Here's how the part is built. I have some questions about the finished solid (model axes, mm). A direction names the side the tool comes from. Round coordinates to 2 decimals unless told otherwise and drop trailing zeros. Loops run counter-clockwise (first coordinate to the right, second up) from the corner with the lowest first, then second, coordinate; pieces in that order, holes last. Notation, with made-up numbers: M -28,-17.5 L 5,-17.5 A29 cw 5,14.5 Z; hole C 71,75 d1. An arc over 180 degrees is marked long. Answer as a JSON object with one key per item and string values.
from build123d import *

# Parameters (mm, degrees)
F0_R     = 5
F1_DEPTH = 30
F2_E1_W  = 3.5025208565
F2_E1_H  = 5
F3_DEPTH = 1


with BuildPart() as f1:
    # F0 (on Right) → F1 (new body)
    with BuildSketch(Plane.YZ):
        Circle(F0_R)
    extrude(amount=F1_DEPTH)

    # F2_E1 (on explicit) → F3 (join)
    with BuildSketch(Plane(origin=(0, 0, 0), x_dir=(0, 0.7071067812, 0.7071067812), z_dir=(0, -0.7071067812, 0.7071067812))):
        with Locations((1.7512604282, 2.5)):
            Rectangle(F2_E1_W, F2_E1_H)
    extrude(amount=F3_DEPTH)


solid = f1.part
Item 1: If I drill on L1, parallel to X at y = -1.75, z = -4; L2, parallel to Z at x = 21, y = -0.25; L3, parallel to Z at x = 6.5, y = 2.75, over which ranges is the centre line in solid material (lowest first)? Write a range as from..to.
Solution:
{"L1": "x = 0..30", "L2": "z = -4.99..4.99", "L3": "z = -4.18..4.18"}
Item 2: I want a section at A-A on z = 2. List the corners of the cut face in (x, y) for me, plus the area to 3 significant figures.
Solution:
{"outline": "M -5,0.59 L 0,0.59 L 0,-4.58 L 30,-4.58 L 30,4.58 L 0,4.58 L 0,2 L -5,2 Z", "area": "282 mm2"}
Item 3: I want a section at D-D on y = 3.75. List the corners of the cut face in (x, z) for me.
Solution:
{"outline": "M 0,-3.31 L 30,-3.31 L 30,3.31 L 0,3.31 Z"}
Item 4: I want a section at C-C on x = 16.5. List the corners of the cut face in (y, z) for me, plus the area to 3 significant figures.
Solution:
{"outline": "C 0,0 d10", "area": "78.5 mm2"}
Item 5: For P1, Ø4, axis at y = -4, z = 2, coming from the -X side, with a flat end and sliding along its axis, tell me the tip position at first contact or that it passes through.
Solution:
{"P1": "stops at x = 0"}
Item 6: I want a section at B-B on y = -3. List the corners of the cut face in (x, z) for me.
Solution:
{"outline": "M 0,-4 L 30,-4 L 30,4 L 0,4 Z"}
Item 7: For faces 1 (the face through (14.79, -1.08, -4.88)), 2 (the face through (-2.535, 0.514, 1.928)), 3 (the face through (-3, 1, 1)), which set-ups out of +Z, -Z, +X, -X, +Y, -Y let a thin tool reach every point of the face, with its end or its side?
Solution:
{"face 1": "+X, -X", "face 2": "+Z, -X, -Y", "face 3": "-Z, -X, +Y"}
